Model file for the job. Use its own axes, mm. Round coordinates to 2 decimals unless told otherwise and drop trailing zeros. Write item = value, one per line. Start each with the question number.
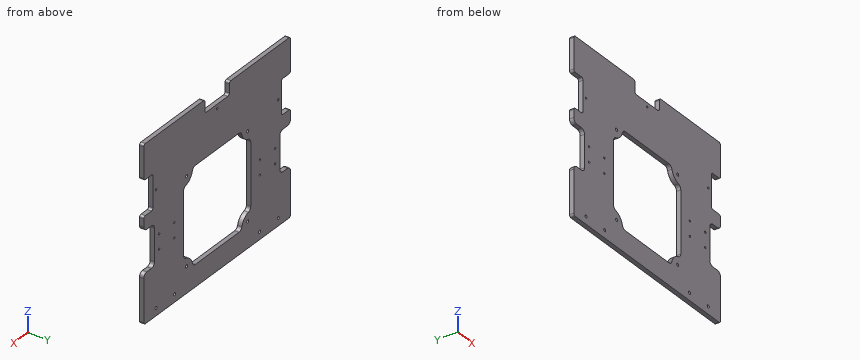
from build123d import *

# Parameters (mm, degrees)
SKETCH2_W                = 304.8
SKETCH2_H                = 254
BASE_DEPTH               = 6.35
SKETCH5_W                = 139.7
SKETCH5_H                = 139.7
FAN_CUTOUT_DEPTH         = 6.35
BOSS_EXTRUDE1_DEPTH      = 6.35
SKETCH8_R                = 2.15265
CUT_EXTRUDE1_DEPTH       = 6.35
FILLET2_R                = 6.35
SKETCH3_W                = 22.225
SKETCH3_H                = 60
WHEEL_CUTOUTS_DEPTH      = 6.35
WHEEL_FILLETS_R          = 6.35
SKETCH4_R                = 1.4732
SKETCH4_W                = 19.05
SKETCH4_H                = 50.8
SKETCH4_W_2              = 50.8
SKETCH4_H_2              = 19.05
ULTRASONIC_CUTOUTS_DEPTH = 6.35
ULTRASONIC_FILLETS_R     = 3.175
FILLET3_R                = 3.175
SKETCH9_R                = 2.15265
CUT_EXTRUDE2_DEPTH       = 6.35
SKETCH10_R               = 1.4732
CUT_EXTRUDE3_DEPTH       = 6.35


with BuildPart() as part:
    # Sketch2 → Base (new body)
    with BuildSketch(Plane(origin=(0, 0, 0), x_dir=(1, 0, 0), z_dir=(0, 1, 0))):
        with Locations((0, -25.4)):
            Rectangle(SKETCH2_W, SKETCH2_H)
    extrude(amount=BASE_DEPTH)

    # Sketch5 → Fan Cutout (cut)
    with BuildSketch(Plane(origin=(0, 6.35, 0), x_dir=(1, 0, 0), z_dir=(0, 1, 0))):
        Rectangle(SKETCH5_W, SKETCH5_H)
    extrude(amount=-FAN_CUTOUT_DEPTH, mode=Mode.SUBTRACT)

    # Sketch7 → Boss-Extrude1 (add)
    with BuildSketch(Plane(origin=(0, 6.35, 0), x_dir=(1, 0, 0), z_dir=(0, 1, 0))):
        with BuildLine():
            Line((-69.85, 50.8), (-69.85, 69.85))
            Line((-69.85, 69.85), (-50.8, 69.85))
            ThreePointArc((-50.8, 69.85), (-56.379615818, 56.379615818), (-69.85, 50.8))
        make_face()
        with BuildLine():
            Line((50.8, 69.85), (69.85, 69.85))
            Line((69.85, 69.85), (69.85, 50.8))
            ThreePointArc((69.85, 50.8), (56.379615818, 56.379615818), (50.8, 69.85))
        make_face()
        with BuildLine():
            Line((-69.85, -50.8), (-69.85, -69.85))
            Line((-69.85, -69.85), (-50.8, -69.85))
            ThreePointArc((-50.8, -69.85), (-56.379615818, -56.379615818), (-69.85, -50.8))
        make_face()
        with BuildLine():
            Line((50.8, -69.85), (69.85, -69.85))
            Line((69.85, -69.85), (69.85, -50.8))
            ThreePointArc((69.85, -50.8), (56.379615818, -56.379615818), (50.8, -69.85))
        make_face()
    extrude(amount=-BOSS_EXTRUDE1_DEPTH)

    # Sketch8 → Cut-Extrude1 (cut)
    with BuildSketch(Plane(origin=(0, 6.35, 0), x_dir=(1, 0, 0), z_dir=(0, 1, 0))):
        with Locations((-63.5, 63.5)):
            Circle(SKETCH8_R)
        with Locations((63.5, 63.5)):
            Circle(SKETCH8_R)
        with Locations((63.5, -63.5)):
            Circle(SKETCH8_R)
        with Locations((-63.5, -63.5)):
            Circle(SKETCH8_R)
    extrude(amount=-CUT_EXTRUDE1_DEPTH, mode=Mode.SUBTRACT)

    # Fillet2
    fillet2_edges = [part.edges().sort_by_distance(p)[0] for p in [
        (-69.85, 3.175, -50.8),
        (-50.8, 3.175, -69.85),
        (50.8, 3.175, -69.85),
        (69.85, 3.175, -50.8),
        (-50.8, 3.175, 69.85),
        (-69.85, 3.175, 50.8),
        (69.85, 3.175, 50.8),
        (50.8, 3.175, 69.85),
    ]]
    fillet(fillet2_edges, radius=FILLET2_R)

    # Sketch3 → Wheel Cutouts (cut)
    with BuildSketch(Plane(origin=(0, 6.35, 0), x_dir=(1, 0, 0), z_dir=(0, 1, 0))):
        with Locations((-141.2875, 0)):
            Rectangle(SKETCH3_W, SKETCH3_H)
        with Locations((141.2875, 0)):
            Rectangle(SKETCH3_W, SKETCH3_H)
    extrude(amount=-WHEEL_CUTOUTS_DEPTH, mode=Mode.SUBTRACT)

    # Wheel Fillets
    wheel_fillets_edges = [part.edges().sort_by_distance(p)[0] for p in [
        (-130.175, 3.175, 30),
        (-130.175, 3.175, -30),
        (-152.4, 3.175, -30),
        (-152.4, 3.175, 30),
        (130.175, 3.175, -30),
        (130.175, 3.175, 30),
        (152.4, 3.175, 30),
        (152.4, 3.175, -30),
    ]]
    fillet(wheel_fillets_edges, radius=WHEEL_FILLETS_R)

    # Sketch4 → Ultrasonic Cutouts (cut)
    with BuildSketch(Plane(origin=(0, 6.35, 0), x_dir=(1, 0, 0), z_dir=(0, 1, 0))):
        with Locations((-127, -76.2)):
            Circle(SKETCH4_R)
        with Locations((127, -76.2)):
            Circle(SKETCH4_R)
        with Locations((0, -127)):
            Circle(SKETCH4_R)
        with Locations((-142.875, -76.2)):
            Rectangle(SKETCH4_W, SKETCH4_H)
        with Locations((142.875, -76.2)):
            Rectangle(SKETCH4_W, SKETCH4_H)
        with Locations((0, -142.875)):
            Rectangle(SKETCH4_W_2, SKETCH4_H_2)
    extrude(amount=-ULTRASONIC_CUTOUTS_DEPTH, mode=Mode.SUBTRACT)

    # Ultrasonic Fillets
    ultrasonic_fillets_edges = [part.edges().sort_by_distance(p)[0] for p in [
        (-133.35, 3.175, 101.6),
        (-133.35, 3.175, 50.8),
        (-152.4, 3.175, 50.8),
        (-152.4, 3.175, 101.6),
        (133.35, 3.175, 50.8),
        (133.35, 3.175, 101.6),
        (152.4, 3.175, 101.6),
        (152.4, 3.175, 50.8),
        (25.4, 3.175, 152.4),
        (25.4, 3.175, 133.35),
        (-25.4, 3.175, 133.35),
        (-25.4, 3.175, 152.4),
    ]]
    fillet(ultrasonic_fillets_edges, radius=ULTRASONIC_FILLETS_R)

    # Fillet3
    fillet3_edges = [part.edges().sort_by_distance(p)[0] for p in [
        (-152.4, 3.175, -101.6),
        (152.4, 3.175, -101.6),
        (152.4, 3.175, 152.4),
        (-152.4, 3.175, 152.4),
    ]]
    fillet(fillet3_edges, radius=FILLET3_R)

    # Sketch9 → Cut-Extrude2 (cut)
    with BuildSketch(Plane(origin=(0, 6.35, 0), x_dir=(1, 0, 0), z_dir=(0, 1, 0))):
        with Locations((-127, 90.4875)):
            Circle(SKETCH9_R)
        with Locations((-88.2, 90.4875)):
            Circle(SKETCH9_R)
        with Locations((88.2, 90.4875)):
            Circle(SKETCH9_R)
        with Locations((127, 90.4875)):
            Circle(SKETCH9_R)
    extrude(amount=-CUT_EXTRUDE2_DEPTH, mode=Mode.SUBTRACT)

    # Sketch10 → Cut-Extrude3 (cut)
    with BuildSketch(Plane(origin=(0, 6.35, 0), x_dir=(1, 0, 0), z_dir=(0, 1, 0))):
        with Locations((-120.625, 10.85)):
            Circle(SKETCH10_R)
        with Locations((-88.875, 10.85)):
            Circle(SKETCH10_R)
        with Locations((-120.625, -10.85)):
            Circle(SKETCH10_R)
        with Locations((-88.875, -10.85)):
            Circle(SKETCH10_R)
        with Locations((88.875, 10.85)):
            Circle(SKETCH10_R)
        with Locations((120.625, 10.85)):
            Circle(SKETCH10_R)
        with Locations((88.875, -10.85)):
            Circle(SKETCH10_R)
        with Locations((120.625, -10.85)):
            Circle(SKETCH10_R)
    extrude(amount=-CUT_EXTRUDE3_DEPTH, mode=Mode.SUBTRACT)


solid = part.part
Item 1: Saw through at A-A, the plane y = 3. Give the number of separate pieces and of enclosed holes in the cut face, then the cut area to 3 significant figures.
Item 2: Probe L1, parallel to X at y = 4.5, z = 10.85 (3 decimals); L2, parallel to Z at x = 127, y = 4.75; L3, parallel to Z at x = 137, y = 5.5. List the from-to ranges inside material, lowest first.
Item 3: Drop flat-ended pins along their axis: pin 1 (3 mm diameter, centred on y = 1.5, z = -4, fed in from +X) (3 decimals); pin 2 (3 mm diameter, centred on y = 4.5, z = 81, fed in from +X). Give the stop position or say it passes through.
Check sheet entries:
q1.separate_pieces = 1
q1.enclosed_holes = 20
q1.area = 53,300 mm2
q2.L1 = -130.175 to -122.098, -119.152 to -90.348, -87.402 to -69.85, 69.85 to 87.402, 90.348 to 119.152, 122.098 to 130.175
q2.L2 = -101.6 to -92.64, -88.33 to 74.73, 77.67 to 152.4
q2.L3 = -101.6 to -30, 30 to 50.8, 101.6 to 152.4
q3.pin_1 = 130.175
q3.pin_2 = 133.35
